The model under review builds one solid part; all positions refer to its coordinate system, in mm. Face numbers are marked on the shaded views. A direction names the side the tool comes from. Coordinates: 2 decimals unless noted, no trailing zeros. Loops run counter-clockwise (first coordinate to the right, second up) from the corner with the lowest first, then second, coordinate; pieces in that order, holes last. Notation, with made-up numbers: M -10,5.25 L 13,5.25 A21 ccw 13,35.25 Z; hole C 5,36 d9. An arc over 180 degrees is marked long. Return JSON: item names as keys, results as strings.
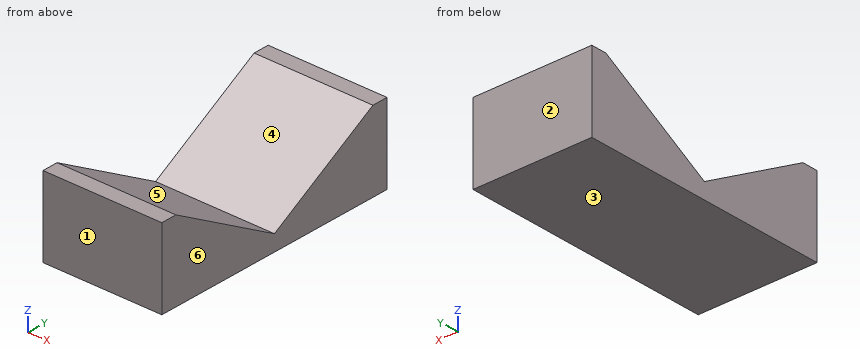
```python
from build123d import *

# Parameters (mm, degrees)
F1_DEPTH = 15


with BuildPart() as f1:
    # F0 (on Right) → F1 (new body)
    with BuildSketch(Plane.YZ):
        Polygon((0, 2), (0, 0), (16, 0), (16, 10), (14, 10), align=None)
    extrude(amount=F1_DEPTH)

    # F2: F1 across face


with BuildPart() as f1_1:
    add(f1.part)
    add(f1.part.mirror(Plane(origin=(7.5, 0, 1), x_dir=(1, 0, 0), z_dir=(0, -1, 0))))


solid = f1_1.part
```
1. Add section A-A on z = 4. Give the boundary of the cut face in (x, y).
Check values:
{"outline": "M 0,-16 L 15,-16 L 15,-3.5 L 0,-3.5 Z; M 0,3.5 L 15,3.5 L 15,16 L 0,16 Z"}
2. Add section B-B on x = 6.75. Give the boundary of the cut face in (y, z), plus the area to 3 significant figures.
Check values:
{"outline": "M -16,0 L 16,0 L 16,10 L 14,10 L 0,2 L -14,10 L -16,10 Z", "area": "208 mm²"}
3. Add section C-C on z = 7. Give the boundary of the cut face in (x, y).
Check values:
{"outline": "M 0,-16 L 15,-16 L 15,-8.75 L 0,-8.75 Z; M 0,8.75 L 15,8.75 L 15,16 L 0,16 Z"}
4. Machinability: for the marked faces 5 and 6, which of the approach directions +Z, -Z, +X, -X, +Y, -Y give a long, thin tool a straight path to every point of the face, cutting with its end or side? Answer none if there is none.
Check values:
{"face 5": "+Z, +X, -X", "face 6": "+Z, -Z, +X, +Y, -Y"}
5. To check wall thickness, follow line 1 (Y direction, x = 8.25, z = 2.25); line 2 (Y direction, x = 2.25, z = 6.75); line 3 (Z direction, x = 12.5, y = -5). State the ranges of each line that lie inside material, in increasing order.
Check values:
{"line 1": "-16 to -0.44, 0.44 to 16", "line 2": "-16 to -8.31, 8.31 to 16", "line 3": "0 to 4.86"}
6. Add section D-D on y = -12.5. Give the boundary of the cut face in (x, z).
Check values:
{"outline": "M 0,0 L 15,0 L 15,9.14 L 0,9.14 Z"}
7. Insertion check: pin 1 Ø3 at (y, z) = (5.5, 2.5) entering from -X; pin 2 Ø1.5 at (x, y) = (4, -9.5) entering from +Z; pin 3 Ø5 at (x, y) = (9.5, -10) entering from +Z. Each pin has a flat end and moves straight along its axis. Give the tip position at first contact, or say it passes through.
Check values:
{"pin 1": "x = 0", "pin 2": "z = 7.86", "pin 3": "z = 9.14"}
8. The part is to be moulded in two halves that separate along Y. For the marked faces 1, 2, 3 and 4, say which applies: released by +Y, released by -Y, zero draft, split by the parting line, or undercut.
Check values:
{"face 1": "released by -Y", "face 2": "released by +Y", "face 3": "zero draft", "face 4": "undercut"}
